Part print with two shaded views. Sizes in mm from the minimum x, y, z corner. Coordinates: 2 decimals unless noted, no trailing zeros. Order: outer loops, then holes, each group sorted by start corner. A loop starts at its lowest first (then second) coordinate and runs counter-clockwise, first axis right, second up.
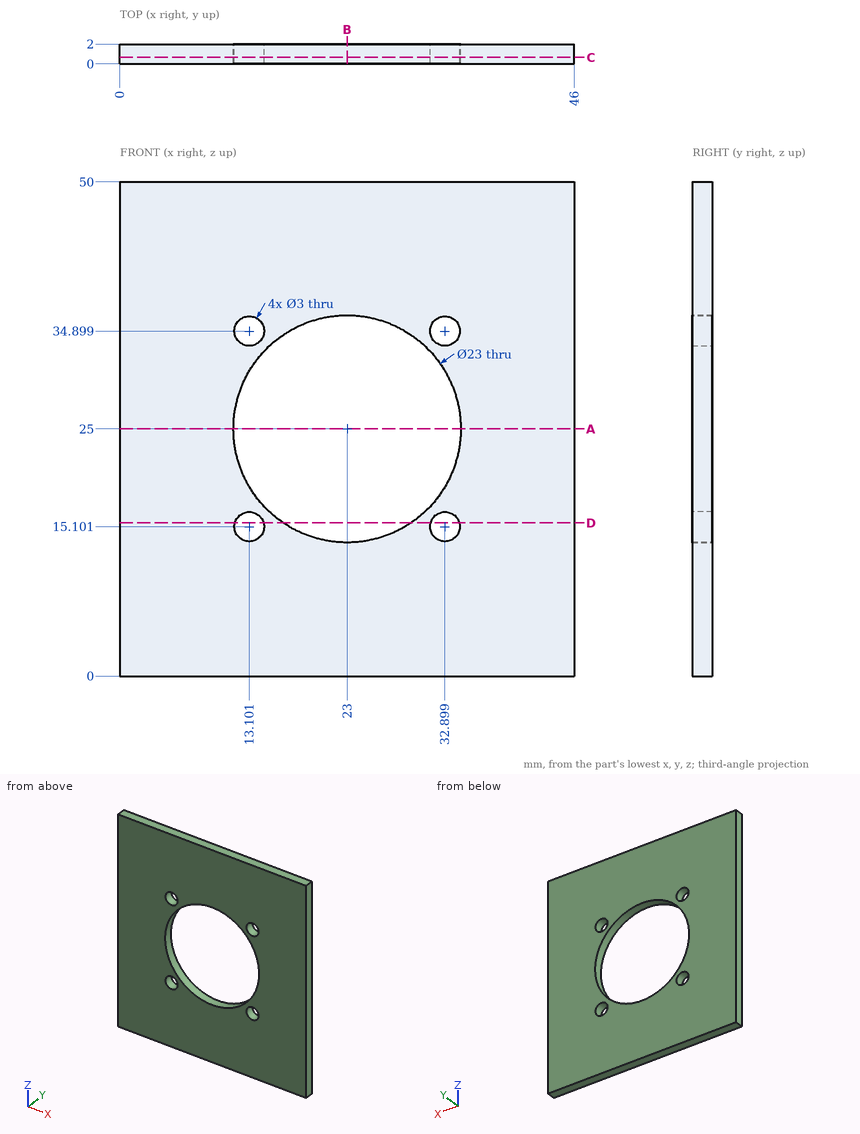
Q1. Cut at B-B on x = 23. Write the cut outline in (y, z).
Results list:
outline: (0, 0) - (2, 0) - (2, 13.5) - (0, 13.5) - close; (0, 36.5) - (2, 36.5) - (2, 50) - (0, 50) - close
Q2. Pin check, flat tip, straight feed: pin 1 Ø2.5 at (x, z) = (13.1, 34.9) entering from -Y. Stop position of the tip, or through.
Results list:
pin 1: passes through
Q3. Cut at D-D on z = 15.5. Write the cut outline in (x, y) (1 decimal).
Results list:
outline: (0, 0) - (11.7, 0) - (11.7, 2) - (0, 2) - close; (14.5, 0) - (16.5, 0) - (16.5, 2) - (14.5, 2) - close; (29.5, 0) - (31.5, 0) - (31.5, 2) - (29.5, 2) - close; (34.3, 0) - (46, 0) - (46, 2) - (34.3, 2) - close
Q4. Wall check: line 1 along X through (y, z) = (1.2, 34); line 2 along Z through (x, y) = (14, 1.55); line 3 along Z through (x, y) = (13, 0.4) (1 decimal). Give the ranges that are in metal, low to high.
Results list:
line 1: x = 0 to 11.9, 14.3 to 15.84, 30.16 to 31.7, 34.1 to 46
line 2: z = 0 to 13.9, 16.3 to 17.84, 32.16 to 33.7, 36.1 to 50
line 3: z = 0 to 13.6, 16.6 to 19.3, 30.7 to 33.4, 36.4 to 50
Q5. Cut at C-C on y = 0.65. Write the cut outline in (x, z), and give its area (3 significant figures).
Results list:
outline: (0, 0) - (46, 0) - (46, 50) - (0, 50) - close; hole circle Ø23 at (23, 25); hole circle Ø3 at (13.1, 15.1); hole circle Ø3 at (13.1, 34.9); hole circle Ø3 at (32.9, 15.1); hole circle Ø3 at (32.9, 34.9)
area: 1,860 mm2
Q6. Cut at A-A on z = 25. Write the cut outline in (x, y).
Results list:
outline: (0, 0) - (11.5, 0) - (11.5, 2) - (0, 2) - close; (34.5, 0) - (46, 0) - (46, 2) - (34.5, 2) - close
